from build123d import *

# Parameters (mm, degrees)
SM_BASE_FLANGE_1_DEPTH = 2
FILLET_1_R             = 5
SKETCH_2_R             = 2.1
CUT_EXTRUDE_1_DEPTH    = 10
SKETCH_3_R             = 2
CUT_EXTRUDE_2_DEPTH    = 10


# Sheet-metal steps are written as plain solids
with BuildPart() as part:
    # Sketch 1 → Базовая кромка1 (new body)
    with BuildSketch(Plane(origin=(0, 0, 0), x_dir=(1, 0, 0), z_dir=(0, 1, 0))):
        with BuildLine():
            Line((-138.290458646, 310.605455598), (-162.69465723, 365.418183057))
            ThreePointArc((-162.69465723, 365.418183057), (0, 400), (162.69465723, 365.418183057))
            Line((162.69465723, 365.418183057), (138.290458646, 310.605455598))
            ThreePointArc((138.290458646, 310.605455598), (0, 340), (-138.290458646, 310.605455598))
        make_face()
    extrude(amount=-SM_BASE_FLANGE_1_DEPTH)

    # Скругление1
    fillet_1_edges = [part.edges().sort_by_distance(p)[0] for p in [
        (-138.290458646, -1, -310.605455598),
        (-162.69465723, -1, -365.418183057),
        (162.69465723, -1, -365.418183057),
        (138.290458646, -1, -310.605455598),
    ]]
    fillet(fillet_1_edges, radius=FILLET_1_R)

    # Эскиз2 → Вырез-Вытянуть1 (cut)
    with BuildSketch(Plane(origin=(0, 0, 0), x_dir=(1, 0, 0), z_dir=(0, 1, 0))):
        with Locations(Location((0, 350, 0), (0, 0, 270))):
            Circle(SKETCH_2_R)
        with Locations(Location((0, 390, 0), (0, 0, 270))):
            Circle(SKETCH_2_R)
    extrude(amount=-CUT_EXTRUDE_1_DEPTH, mode=Mode.SUBTRACT)

    # Эскиз3 → Вырез-Вытянуть2 (cut)
    with BuildSketch(Plane(origin=(0, 0, 0), x_dir=(1, 0, 0), z_dir=(0, 1, 0))):
        with Locations(Location((-135.741676964, 317.173764891, 0), (0, 0, 270))):
            Circle(SKETCH_3_R)
        with Locations(Location((-156.080374798, 362.85522816, 0), (0, 0, 270))):
            Circle(SKETCH_3_R)
        with Locations(Location((135.741676964, 317.173764891, 0), (0, 0, 270))):
            Circle(SKETCH_3_R)
        with Locations(Location((156.080374798, 362.85522816, 0), (0, 0, 270))):
            Circle(SKETCH_3_R)
    extrude(amount=-CUT_EXTRUDE_2_DEPTH, mode=Mode.SUBTRACT)


solid = part.part
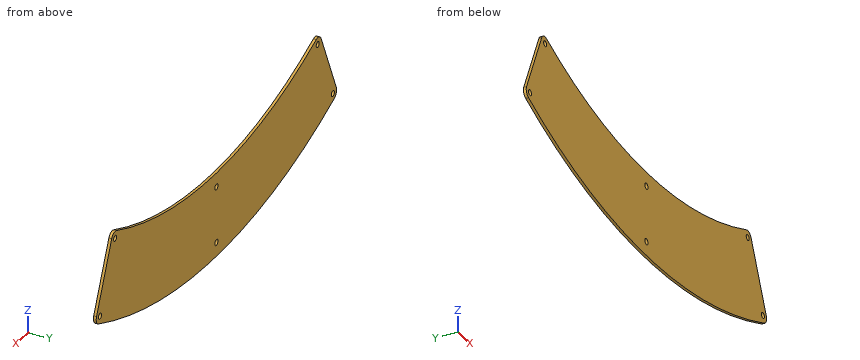
Geometry check sheet. Reference: the model listing, model coordinates, mm. Round coordinates to 2 decimals unless told otherwise and drop trailing zeros. Loops run counter-clockwise (first coordinate to the right, second up) from the corner with the lowest first, then second, coordinate; pieces in that order, holes last. Notation, with made-up numbers: (51, 28.5) - (80, 28.5) arc R26 cw to (80, 49.5) - close; hole circle Ø8 at (56.5, -29.5). An arc over 180 degrees is marked (long way). One line per question, with ' | ' between items. Start each with the question number.
1. Scan lines: line 1 (X direction, y = -1.5, z = -350); line 2 (X direction, y = -1.2, z = -342); line 3 (Z direction, x = 92, y = -1.55). Record each from-to range of solid material in increasing order. Write a range as [from, to].
2. Cross-section at C-C on x = 67. Record the cut outline in (y, z).
3. Cross-section at B-B on x = 23.5. Record the cut outline in (y, z), then the cut area to 3 significant figures.
4. Cross-section at A-A on y = -0.6. Record the cut outline in (x, z), then the cut area to 3 significant figures.
Taken from the geometry:
1) line 1: [-155.83, -2.1], [2.1, 155.83] | line 2: [-152.27, 152.27] | line 3: [-389.28, -327.32]
2) outline: (-2, -394.35) - (0, -394.35) - (0, -333.33) - (-2, -333.33) - close
3) outline: (-2, -399.31) - (0, -399.31) - (0, -339.19) - (-2, -339.19) - close | area: 120 mm²
4) outline: (-160.65, -360.82) arc R5 ccw to (-158.06, -367.45) arc R400 ccw to (158.06, -367.45) arc R5 ccw to (160.65, -360.82) - (140.31, -315.14) arc R5 ccw to (133.77, -312.58) arc R340 cw to (-133.77, -312.58) arc R5 ccw to (-140.31, -315.14) - close; hole circle Ø4 at (-156.08, -362.86); hole circle Ø4 at (-135.74, -317.17); hole circle Ø4.2 at (0, -390); hole circle Ø4.2 at (0, -350); hole circle Ø4 at (135.74, -317.17); hole circle Ø4 at (156.08, -362.86) | area: 18,500 mm²
